Solid Edge part; units mm, degrees
sketch "Sketch1" plane through (0, 0, 0) normal (0, -1, 0) x (1, 0, 0)
  line L0 (8.5, 0.45) -> (-7, 0.625)
  line L1 (-7, 0.625) -> (-20.5, 0.5)
  line L2 (-20.5, 0.5) -> (-22.5, 0.45)
  line L3 (-22.5, 0.45) -> (-22.5, 0)
  line L4 (-20.5, 0.05) -> (-22.5, 0)
  line L5 (-20.5, 0.05) -> (-7, 0.175)
  line L6 (-7, 0.175) -> (8.5, 0)
  line L7 (8.5, 0) -> (22.5, 0)
  line L8 (22.5, 0) -> (22.5, 0.45)
  line L9 (22.5, 0.45) -> (8.5, 0.45)
extrude "Protrusion1" add sketch "Sketch1" along normal mid plane 3
sketch "Sketch2" plane through (15.5, 0, 0.45) normal (0, 0, 1) x (0, 1, 0)
  circle A0 centre (0, -2.5) radius 1
extrude "ExtrudedCutout_3" cut sketch "Sketch2" against normal blind 0.45
sketch "Sketch3" plane through (15.5, 0, 0.45) normal (0, 0, 1) x (0, 1, 0)
  circle A0 centre (0, -5.5) radius 1
extrude "ExtrudedCutout_4" cut sketch "Sketch3" against normal blind 0.45
Verification items for the finished model (mm, model axes). Give positions to 0.01 mm unless a question says otherwise; leave off trailing zeros. Loops run counter-clockwise (first coordinate to the right, second up) from the corner with the lowest first, then second, coordinate; pieces in that order, holes last.
1) Draft check along X on faces 1 (the cylindrical face through (18.976, -0.217, 0.228)), 2 (the cylindrical face through (21.976, -0.217, 0.228)), 3 (the flat face through (14, 0, 0)). Enter one of: pulls with the +X half, pulls with the -X half, needs draft (parallel to the pull), parting line crosses it, or undercut.
2) Depth check by flat-ended pin: pin 1 Ø1.5 at (x, y) = (3.5, 0) entering from -Z. Enter the tip coordinate at first touch or a pass-through.
3) Sectioned sample at A-A, the plane x = 18. Enter the section's corners in (y, z), then the cut area to 3 significant figures.
4) Sectioned sample at C-C, the plane x = -10.5. Enter the section's corners in (y, z).
5) Thickness scan on line 1 along X through (y, z) = (0, 0.3); line 2 along Y through (x, z) = (18, 0.25); line 3 along Z through (x, y) = (-7, -0.1) (3 decimals). Record the ranges inside material, lowest first.
6) Sectioned sample at B-B, the plane y = 0. Enter the section's corners in (x, z) (3 decimals).
Answers:
1. face 1: undercut
1. face 2: undercut
1. face 3: needs draft
2. pin 1: stops at z = 0.05
3. outline: (-1.5, 0) - (-1, 0) - (-1, 0.45) - (-1.5, 0.45) - close; (1, 0) - (1.5, 0) - (1.5, 0.45) - (1, 0.45) - close
3. area: 0.450 mm2
4. outline: (-1.5, 0.14) - (1.5, 0.14) - (1.5, 0.59) - (-1.5, 0.59) - close
5. line 1: x = -22.5 to 17, 19 to 20, 22 to 22.5
5. line 2: y = -1.5 to -1, 1 to 1.5
5. line 3: z = 0.175 to 0.625
6. outline: (-22.5, 0) - (-20.5, 0.05) - (-7, 0.175) - (8.5, 0) - (17, 0) - (17, 0.45) - (8.5, 0.45) - (-7, 0.625) - (-20.5, 0.5) - (-22.5, 0.45) - close; (19, 0) - (20, 0) - (20, 0.45) - (19, 0.45) - close; (22, 0) - (22.5, 0) - (22.5, 0.45) - (22, 0.45) - close
